Part model, mm, in its own coordinate system. A direction names the side the tool comes from. Round coordinates to 2 decimals unless told otherwise and drop trailing zeros. Loops run counter-clockwise (first coordinate to the right, second up) from the corner with the lowest first, then second, coordinate; pieces in that order, holes last.
from build123d import *

# Parameters (mm, degrees)
F1_DEPTH = 10
F2_R     = 4.99999
F3_R     = 2
F4_DEPTH = 2
F5_R     = 2
F6_DEPTH = 2


# Not quite as in the source:
# - a fillet or chamfer is up to 0.001 mm smaller than in the source, because OpenCascade refuses the exact size


with BuildPart() as f1:
    # F0 (on Top) → F1 (new body)
    with BuildSketch(Plane.XY):
        Polygon((-5, 4), (-4.1339745962, 5.5), (-5.8660254038, 5.5), align=None)
        Polygon((-26.857039656, -8.0272581187), (-9.163588619, -4.7194203959), (-9.5311261437, -2.7534813918), (-27.2245771808, -6.0613191145), align=None)
        with BuildLine():
            ThreePointArc((-3.4370598373, -4.2937884991), (-2.75, -4.7631397208), (-2, -5.123475383))
            Line((-2, -5.123475383), (-2, -3.4641016151))
            Line((-2, -3.4641016151), (-3.4370598373, -4.2937884991))
        make_face()
        with BuildLine():
            ThreePointArc((-0.8296868839, -5.4370598373), (0, -5.5), (0.8296868839, -5.4370598373))
            Line((0.8296868839, -5.4370598373), (0, -4))
            Line((0, -4), (-0.8296868839, -5.4370598373))
        make_face()
        with BuildLine():
            ThreePointArc((2, -5.123475383), (2.75, -4.7631397208), (3.4370598373, -4.2937884991))
            Line((3.4370598373, -4.2937884991), (2, -3.4641016151))
            Line((2, -3.4641016151), (2, -5.123475383))
        make_face()
        with BuildLine():
            ThreePointArc((4.2937884991, -3.4370598373), (4.7631397208, -2.75), (5.123475383, -2))
            Line((5.123475383, -2), (3.4641016151, -2))
            Line((3.4641016151, -2), (4.2937884991, -3.4370598373))
        make_face()
        with BuildLine():
            ThreePointArc((5.4370598373, -0.8296868839), (5.5, 0), (5.4370598373, 0.8296868839))
            Line((5.4370598373, 0.8296868839), (4, 0))
            Line((4, 0), (5.4370598373, -0.8296868839))
        make_face()
        with BuildLine():
            Line((0, 4), (0.8296868839, 5.4370598373))
            ThreePointArc((0.8296868839, 5.4370598373), (0.416035392, 5.4842423864), (0, 5.5))
            Line((0, 5.5), (0, 4))
        make_face()
        with BuildLine():
            ThreePointArc((0, 5.5), (0.416035392, 5.4842423864), (0.8296868839, 5.4370598373))
            Line((0.8296868839, 5.4370598373), (0.8660254038, 5.5))
            Line((0.8660254038, 5.5), (0, 5.5))
        make_face()
        with BuildLine():
            Line((0, 4), (0, 5.5))
            ThreePointArc((0, 5.5), (-0.416035392, 5.4842423864), (-0.8296868839, 5.4370598373))
            Line((-0.8296868839, 5.4370598373), (0, 4))
        make_face()
        with BuildLine():
            Line((-2, 4.8660254038), (-1.8110659829, 5.1932687207))
            ThreePointArc((-1.8110659829, 5.1932687207), (-1.9058525019, 5.1592369824), (-2, 5.123475383))
            Line((-2, 5.123475383), (-2, 4.8660254038))
        make_face()
        with BuildLine():
            Line((-2, 4.8660254038), (-2, 5.123475383))
            ThreePointArc((-2, 5.123475383), (-2.4559554031, 4.9212074797), (-2.8917104606, 4.6784624196))
            Line((-2.8917104606, 4.6784624196), (-2.5, 4))
            Line((-2.5, 4), (-2, 4.8660254038))
        make_face()
        with BuildLine():
            ThreePointArc((-9.163588619, -4.7194203959), (-6.8106363862, -4.7920452574), (-4.7035733226, -5.8417803792))
            ThreePointArc((-4.7035733226, -5.8417803792), (-6.0524247462, -4.4292386131), (-6.9908223073, -2.7163216797))
            ThreePointArc((-6.9908223073, -2.7163216797), (-8.2625591256, -2.6265549538), (-9.5311261437, -2.7534813918))
            Line((-9.5311261437, -2.7534813918), (-9.163588619, -4.7194203959))
        make_face()
        with BuildLine():
            Line((-4.6842221141, -1.9200455203), (-4.9155419039, -2.4672753781))
            ThreePointArc((-4.9155419039, -2.4672753781), (-4.7096941165, -2.8405600379), (-4.4755547297, -3.196781172))
            Line((-4.4755547297, -3.196781172), (-4.6842221141, -1.9200455203))
        make_face()
        with BuildLine():
            Line((-4.6842221141, -1.9200455203), (-5.0512472947, -2.175982713))
            ThreePointArc((-5.0512472947, -2.175982713), (-4.9855224988, -2.3226203765), (-4.9155419039, -2.4672753781))
            Line((-4.9155419039, -2.4672753781), (-4.6842221141, -1.9200455203))
        make_face()
        with BuildLine():
            ThreePointArc((-0.8296868839, 5.4370598373), (-0.416035392, 5.4842423864), (0, 5.5))
            Line((0, 5.5), (-0.8660254038, 5.5))
            Line((-0.8660254038, 5.5), (-0.8296868839, 5.4370598373))
        make_face()
        with BuildLine():
            Line((-5.0512472947, -2.175982713), (-6.104954117, -2.9107627231))
            ThreePointArc((-6.104954117, -2.9107627231), (-5.6640980624, -3.0507217811), (-5.2327078262, -3.2175901813))
            Line((-5.2327078262, -3.2175901813), (-4.9155419039, -2.4672753781))
            ThreePointArc((-4.9155419039, -2.4672753781), (-4.9855224988, -2.3226203765), (-5.0512472947, -2.175982713))
        make_face()
        with BuildLine():
            ThreePointArc((-2, 5.123475383), (-1.9058525019, 5.1592369824), (-1.8110659829, 5.1932687207))
            Line((-1.8110659829, 5.1932687207), (-1.6339745962, 5.5))
            Line((-1.6339745962, 5.5), (-3.3660254038, 5.5))
            Line((-3.3660254038, 5.5), (-2.8917104606, 4.6784624196))
            ThreePointArc((-2.8917104606, 4.6784624196), (-2.4559554031, 4.9212074797), (-2, 5.123475383))
        make_face()
        with BuildLine():
            Line((-4.9155419039, -2.4672753781), (-5.2327078262, -3.2175901813))
            ThreePointArc((-5.2327078262, -3.2175901813), (-4.8124241684, -3.4107332523), (-4.404845606, -3.629416389))
            Line((-4.404845606, -3.629416389), (-4.4755547297, -3.196781172))
            ThreePointArc((-4.4755547297, -3.196781172), (-4.7096941165, -2.8405600379), (-4.9155419039, -2.4672753781))
        make_face()
        with BuildLine():
            ThreePointArc((0.8296868839, 5.4370598373), (1.4235047481, 5.3125920446), (2, 5.123475383))
            Line((2, 5.123475383), (2, 3.4641016151))
            Line((2, 3.4641016151), (3.4370598373, 4.2937884991))
            ThreePointArc((3.4370598373, 4.2937884991), (3.8890872965, 3.8890872965), (4.2937884991, 3.4370598373))
            Line((4.2937884991, 3.4370598373), (3.4641016151, 2))
            Line((3.4641016151, 2), (5.123475383, 2))
            ThreePointArc((5.123475383, 2), (5.3125920446, 1.4235047481), (5.4370598373, 0.8296868839))
            ThreePointArc((5.4370598373, 0.8296868839), (5.5, 0), (5.4370598373, -0.8296868839))
            ThreePointArc((5.4370598373, -0.8296868839), (5.3125920446, -1.4235047481), (5.123475383, -2))
            ThreePointArc((5.123475383, -2), (4.7631397208, -2.75), (4.2937884991, -3.4370598373))
            ThreePointArc((4.2937884991, -3.4370598373), (3.8890872965, -3.8890872965), (3.4370598373, -4.2937884991))
            ThreePointArc((3.4370598373, -4.2937884991), (2.75, -4.7631397208), (2, -5.123475383))
            ThreePointArc((2, -5.123475383), (1.4235047481, -5.3125920446), (0.8296868839, -5.4370598373))
            ThreePointArc((0.8296868839, -5.4370598373), (0, -5.5), (-0.8296868839, -5.4370598373))
            ThreePointArc((-0.8296868839, -5.4370598373), (-1.4235047481, -5.3125920446), (-2, -5.123475383))
            ThreePointArc((-2, -5.123475383), (-2.75, -4.7631397208), (-3.4370598373, -4.2937884991))
            ThreePointArc((-3.4370598373, -4.2937884991), (-3.4431769685, -4.2888847459), (-3.4492871033, -4.2839722781))
            ThreePointArc((-3.4492871033, -4.2839722781), (-3.9144118435, -3.9382205471), (-4.404845606, -3.629416389))
            ThreePointArc((-4.404845606, -3.629416389), (-4.8124241684, -3.4107332523), (-5.2327078262, -3.2175901813))
            ThreePointArc((-5.2327078262, -3.2175901813), (-5.6640980624, -3.0507217811), (-6.104954117, -2.9107627231))
            ThreePointArc((-6.104954117, -2.9107627231), (-6.544946362, -2.800139211), (-6.9908223073, -2.7163216797))
            ThreePointArc((-6.9908223073, -2.7163216797), (-6.0524247462, -4.4292386131), (-4.7035733226, -5.8417803792))
            ThreePointArc((-4.7035733226, -5.8417803792), (7.0733073185, -2.493656668), (0, 7.5))
            Line((0, 7.5), (-27.3435036541, 7.5))
            Line((-27.3435036541, 7.5), (-27.3435036541, 5.5))
            Line((-27.3435036541, 5.5), (-5.8660254038, 5.5))
            Line((-5.8660254038, 5.5), (-4.1339745962, 5.5))
            Line((-4.1339745962, 5.5), (-3.3660254038, 5.5))
            Line((-3.3660254038, 5.5), (-1.6339745962, 5.5))
            Line((-1.6339745962, 5.5), (-0.8660254038, 5.5))
            Line((-0.8660254038, 5.5), (0, 5.5))
            Line((0, 5.5), (0.8660254038, 5.5))
            Line((0.8660254038, 5.5), (0.8296868839, 5.4370598373))
        make_face()
    extrude(amount=F1_DEPTH)

    # F2 (radius 5 in the source; OpenCascade refuses exactly that, so slightly less here)
    f2_edges = [f1.edges().sort_by_distance(p)[0] for p in [
        (-27.343504, 6.5, 10),
        (-27.343504, 6.5, 0),
        (-27.040808, -7.044289, 0),
        (-27.040808, -7.044289, 10),
    ]]
    fillet(f2_edges, radius=F2_R)

    # F3 (on face) → F4 (cut)
    with BuildSketch(Plane(origin=(0.5430486336, -2.9047387492, 0), x_dir=(0.9829695021, 0.1837687624, 0), z_dir=(0.1837687624, -0.9829695021, 0))):
        with Locations((-17.8748101871, 5)):
            Circle(F3_R)
    extrude(amount=-F4_DEPTH, mode=Mode.SUBTRACT)

    # F5 (on face) → F6 (cut)
    with BuildSketch(Plane(origin=(0, 7.5, 0), x_dir=(-1, 0, 0), z_dir=(0, 1, 0))):
        with Locations((17.3435036541, 5)):
            Circle(F5_R)
    extrude(amount=-F6_DEPTH, mode=Mode.SUBTRACT)


solid = f1.part
1) Tool access for faces 1 (the face through (-25.637, -6.796, 1.504)), 2 (the face through (-2, -4, 5)), 3 (the face through (3.885, 2.729, 4.93)): list every direction of +Z, -Z, +X, -X, +Y, -Y with a clear straight run to the whole face (end or side of a thin tool).
Values:
face 1: -Z, -X, -Y
face 2: +Z, -Z
face 3: +Z, -Z, -X
2) Slice it at A-A, the plane x = -8.5. Give the cut face in (y, z).
Values:
outline: (-4.64, 0) - (-2.63, 0) - (-2.63, 10) - (-4.64, 10) - close; (5.5, 0) - (7.5, 0) - (7.5, 10) - (5.5, 10) - close
3) Drop flat-ended pins along their axis: pin 1 Ø1.3 at (y, z) = (4, 3) entering from -X; pin 2 Ø0.5 at (y, z) = (-4.5, 4) entering from +X; pin 3 Ø0.5 at (x, z) = (4, 7) entering from +Y. Give the stop position or say it passes through.
Values:
pin 1: stops at x = -5.38
pin 2: stops at x = 6.18
pin 3: stops at y = 6.5
4) Slice it at B-B, the plane z = 4.25. Give the number of separate pieces and of enclosed holes in the cut face, then the cut area to 3 significant figures.
Values:
separate pieces: 3
enclosed holes: 0
area: 150 mm2
5) Wall check: line 1 along Y through (x, z) = (-22, 5.25); line 2 along Y through (x, z) = (-21.5, 7.75); line 3 along X through (y, z) = (-2.5, 6.75). Give the ranges that are in metal, low to high.
Values:
line 1: y = -7.12 to -5.08, 5.5 to 7.5
line 2: y = -7.03 to -4.99, 5.5 to 7.5
line 3: x = -5.52 to -4.59, 3.75 to 7.07
6) Slice it at D-D, the plane x = -20.5. Give the cut face in (y, z).
Values:
outline: (-6.84, 0) - (-4.8, 0) - (-4.8, 10) - (-6.84, 10) - close; (5.5, 0) - (7.5, 0) - (7.5, 10) - (5.5, 10) - close
7) Mould opens along Z. For faces 4 (the face through (-7, -3, 0)), 5 (the face through (2, 4, 5)), 6 (the face through (-19.17, -5.59, 5.09)) say: released by +Z, released by -Z, zero draft, split by the parting line, or undercut.
Values:
face 4: released by -Z
face 5: zero draft
face 6: undercut
